```python
from build123d import *

# Parameters (mm, degrees)
F0_R     = 10
F1_DEPTH = 20
F2_R     = 3
F4_D     = 10


with BuildPart() as f1:
    # F0 (on Front) → F1 (new body)
    with BuildSketch(Plane.XZ):
        Polygon((-40, 5), (-40, 0), (40, 0), (40, 5), (20, 5), (20, 35), (-20, 35), (-20, 5), align=None)
        with Locations((0, 20)):
            Circle(F0_R, mode=Mode.SUBTRACT)
    extrude(amount=F1_DEPTH)

    # F2
    f2_edges = [f1.edges().sort_by_distance(p)[0] for p in [
        (20, -10, 35),
        (20, -10, 5),
        (-20, -10, 35),
        (-20, -10, 5),
    ]]
    fillet(f2_edges, radius=F2_R)

    # F4 (through all)
    with Locations(Plane(origin=(0, 0, 0), x_dir=(1, 0, 0), z_dir=(0, 0, -1))):
        with Locations((-30.768288, 10), (29.231712, 10)):
            Hole(F4_D / 2)


solid = f1.part
```
Could you check a few things on this model? Use its own coordinates, in mm. A direction names the side the tool comes from. Round coordinates to 2 decimals unless told otherwise and drop trailing zeros. Write each loop counter-clockwise with the first axis right and the second up, starting at its lowest first coordinate (ties: lowest second). Pieces come first, ordered by that corner, then holes. Notation, with made-up numbers: M 63.5,79.5 L 68.5,79.5 A11 ccw 68.5,96.5 Z; hole C 12.5,80.25 d11. An arc over 180 degrees is marked long. Answer in a Markdown table with one row per item. Add a question column.
Q1. If I drill on line 1 (X direction, y = -13.75, z = 4); line 2 (Z direction, x = 0, y = -13); line 3 (Y direction, x = 26, z = 4), over which ranges is the centre line in solid material (lowest first)? Write a range as from..to.
Q2. Imagine slicing it at C-C (x = -28). Please give me the cut outline in (y, z), then the cut area to 3 significant figures.
Q3. Imagine slicing it at D-D (y = -18.25). Please give me the cut outline in (x, z), then the cut area to 3 significant figures.
Q4. On a 3-axis mill with a long thin cutter (end or side, diameter ignored), from which of +Z, -Z, +X, -X, +Y, -Y can I reach the whole of each face in a straight line? I mean faces 4 (the flat face through (20, -10, 20)), 5 (the flat face through (-9, 0, 14)), 6 (the flat face through (-33, -5, 5)). Say none if no direction works.
Q5. Imagine slicing it at A-A (y = -10). Please give me the cut outline in (x, z), then the cut area to 3 significant figures.
Q6. Imagine slicing it at B-B (z = 20). Please give me the cut outline in (x, y).
Q7. If we mould it in two halves opening along Y, with no side actions, what happens to faces 1 (the cylindrical face through (-19.14, -10.14, 34.1)), 2 (the flat face through (-9, -20, 14)), 3 (the cylindrical face through (29.883, -14.957, 2.535))? For each: +Y half, -Y half, draft (parallel to the pull), parting line (faces both ways), or undercut.
Q8. Will these pins go through, and if not, where does the flat tip stop? pin 1 Ø6 at (x, y) = (30.5, -7.5) entering from +Z; pin 2 Ø3 at (y, z) = (-6, 23.5) entering from +X; pin 3 Ø6 at (y, z) = (-8, 22.5) entering from -X.
Values:
| question | item | result |
|---|---|---|
| 1 | line 1 | -40..-34.08, -27.46..25.92, 32.54..40 |
| 1 | line 2 | 0..10, 30..35 |
| 1 | line 3 | -20..-13.82, -6.18..0 |
| 2 | outline | M -20,0 L -14.16,0 L -14.16,5 L -20,5 Z; M -5.84,0 L 0,0 L 0,5 L -5.84,5 Z |
| 2 | area | 58.4 mm^2 |
| 3 | outline | M -40,0 L 40,0 L 40,5 L 23,5 A3 cw 20,8 L 20,32 A3 ccw 17,35 L -17,35 A3 ccw -20,32 L -20,8 A3 cw -23,5 L -40,5 Z; hole C 0,20 d20 |
| 3 | area | 1,290 mm^2 |
| 4 | face 4 | +Z, +X, +Y, -Y |
| 4 | face 5 | +Z, -Z, +X, -X, +Y |
| 4 | face 6 | +Z, -X, +Y, -Y |
| 5 | outline | M -40,0 L -35.77,0 L -35.77,5 L -40,5 Z; M -25.77,0 L 24.23,0 L 24.23,5 L 23,5 A3 cw 20,8 L 20,32 A3 ccw 17,35 L -17,35 A3 ccw -20,32 L -20,8 A3 cw -23,5 L -25.77,5 Z; M 34.23,0 L 40,0 L 40,5 L 34.23,5 Z; hole C 0,20 d20 |
| 5 | area | 1,190 mm^2 |
| 6 | outline | M -20,-20 L -10,-20 L -10,0 L -20,0 Z; M 10,-20 L 20,-20 L 20,0 L 10,0 Z |
| 7 | face 1 | draft |
| 7 | face 2 | -Y half |
| 7 | face 3 | undercut |
| 8 | pin 1 | z = 5 |
| 8 | pin 2 | x = 20 |
| 8 | pin 3 | x = -20 |
